Design review of the part shown in the three views and the two pictorial views. Dimensions are in mm from the part's minimum x, y and z. A direction names the side the tool comes from. Coordinates: 2 decimals unless noted, no trailing zeros. Write each loop counter-clockwise with the first axis right and the second up, starting at its lowest first coordinate (ties: lowest second). Pieces come first, ordered by that corner, then holes. Notation, with made-up numbers: (-24.5, -39.75) -> (-4.5, -39.75) arc R16 cw to (-4.5, -23.75) -> close; hole circle Ø9 at (-23.5, -37.75). An arc over 180 degrees is marked (long way). Write each question's results on one line, items separated by ' | '.
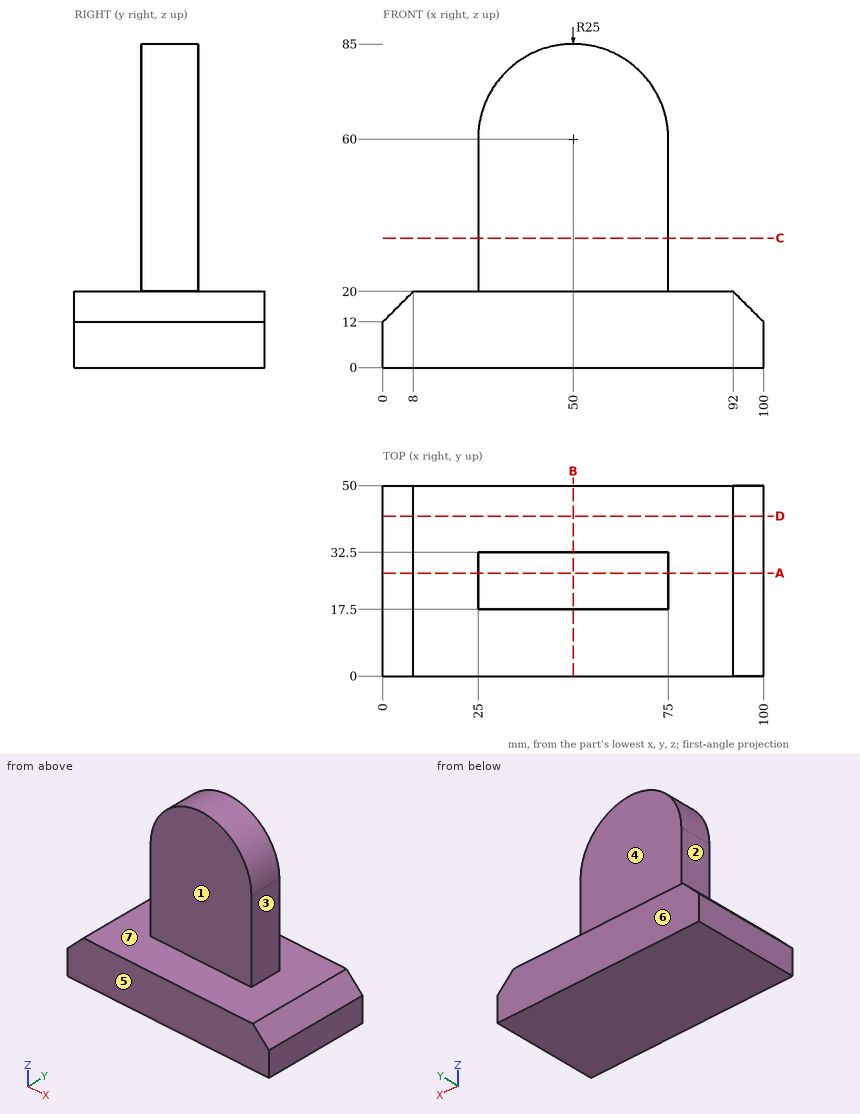
Q1. Add section C-C (z = 34). Write out the cut boundary in (x, y).
Solution:
outline: (25, 17.5) -> (75, 17.5) -> (75, 32.5) -> (25, 32.5) -> close
Q2. Add section A-A (y = 27). Write out the cut boundary in (x, z).
Solution:
outline: (0, 0) -> (100, 0) -> (100, 12) -> (92, 20) -> (75, 20) -> (75, 60) arc R25 ccw to (25, 60) -> (25, 20) -> (8, 20) -> (0, 12) -> close
Q3. Clearance check with flat-ended pins moving along their axes: P1, Ø8, axis at x = 28.5, z = 48, coming from the +Y side; P2, Ø2, axis at x = 52.5, z = 25.5, coming from the -Y side; P3, Ø10, axis at y = 31.5, z = 20, coming from the +X side. State where each tip first meets the part, or that it passes through.
Solution:
P1: y = 32.5 | P2: y = 17.5 | P3: x = 97
Q4. Add section B-B (x = 50). Write out the cut boundary in (y, z), plus the area to 4 significant figures.
Solution:
outline: (0, 0) -> (50, 0) -> (50, 20) -> (32.5, 20) -> (32.5, 85) -> (17.5, 85) -> (17.5, 20) -> (0, 20) -> close | area: 1,975 mm²
Q5. Machinability: for the marked faces 1, 2, 3 and 4, which of the approach directions +Z, -Z, +X, -X, +Y, -Y give a long, thin tool a straight path to every point of the face, cutting with its end or side? Answer none if there is none.
Solution:
face 1: +Z, +X, -X, -Y | face 2: +Z, -X, +Y, -Y | face 3: +Z, +X, +Y, -Y | face 4: +Z, +X, -X, +Y
Q6. Add section D-D (y = 42). Write out the cut boundary in (x, z).
Solution:
outline: (0, 0) -> (100, 0) -> (100, 12) -> (92, 20) -> (8, 20) -> (0, 12) -> close
Q7. Draft analysis for pull direction Y (two halves, no side actions). For the marked faces 5, 6 and 7, state which applies: pulls with the +Y half, pulls with the -Y half, needs draft (parallel to the pull), parting line crosses it, or undercut.
Solution:
face 5: pulls with the -Y half | face 6: pulls with the +Y half | face 7: needs draft
Q8. For line 1 (Y direction, x = 49, z = 69.5); line 2 (Z direction, x = 57, y = 35); line 3 (X direction, y = 29.5, z = 38), list the stretches that pass through material, from the lowest coordinate up. Write a range as from..to.
Solution:
line 1: 17.5..32.5 | line 2: 0..20 | line 3: 25..75
